CAD build for the part. Positions are in the model's coordinates, mm. Coordinates: 2 decimals unless noted, no trailing zeros. Loops run counter-clockwise (first coordinate to the right, second up) from the corner with the lowest first, then second, coordinate; pieces in that order, holes last. Notation, with made-up numbers: (32, -31.5) -> (79, -31.5) arc R14 ccw to (79, -14.5) -> close; hole circle Ø6 at (54.25, 51). An arc over 180 degrees is marked (long way). Write item = value, one per line. Start each with the question number.
(1) Band-saw the part on A-A (x = 95.45). Write the cut outline in (y, z) (3 decimals).
(2) Drill centre lines: line 1 (X direction, y = -3.75, z = 15); line 2 (Z direction, x = 95.45, y = -2.75); line 3 (Z direction, x = -50, y = -7.5). Where is each one in solid material? Low to high. Write a range as from..to.
(3) Flat gauge pin, fed straight in: P1, Ø6, axis at x = -81, z = -16.5, coming from the +Y side. Where does the tip first touch, or does it go through?
```python
from build123d import *

# Parameters (mm, degrees)
SKETCH1_W             = 240.9
SKETCH1_H             = 50.8
BOSS_EXTRUDE1_DEPTH   = 9.525
M3X0_5_TAPPED_HOLE1_D = 2.5
M5_CLEARANCE_HOLE1_D  = 5.5


with BuildPart() as part:
    # Sketch1 → Boss-Extrude1 (new body)
    with BuildSketch(Plane(origin=(0, 0, 0), x_dir=(1, 0, 0), z_dir=(0, 1, 0))):
        Rectangle(SKETCH1_W, SKETCH1_H)
    extrude(amount=-BOSS_EXTRUDE1_DEPTH)

    # M3x0.5 Tapped Hole1 (through all)
    with Locations(Plane(origin=(0, 0, 0), x_dir=(1, 0, 0), z_dir=(0, 1, 0))):
        with Locations((-50, 15), (-50, -15), (50, -15), (50, 15)):
            Hole(M3X0_5_TAPPED_HOLE1_D / 2)

    # M5 Clearance Hole1 (through all)
    with Locations(Plane(origin=(0, 0, 0), x_dir=(1, 0, 0), z_dir=(0, 1, 0))):
        with Locations((95.45, 15), (-95.45, 15), (-95.45, -15), (95.45, -15)):
            Hole(M5_CLEARANCE_HOLE1_D / 2)


solid = part.part
```
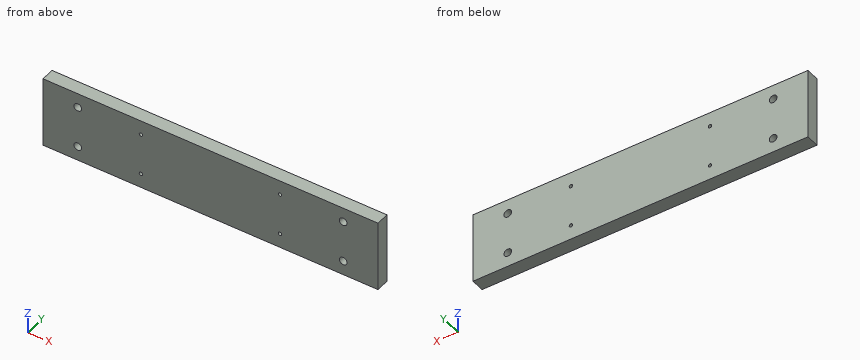
Findings below:
q1.outline = (-9.525, -25.4) -> (0, -25.4) -> (0, -17.75) -> (-9.525, -17.75) -> close; (-9.525, -12.25) -> (0, -12.25) -> (0, 12.25) -> (-9.525, 12.25) -> close; (-9.525, 17.75) -> (0, 17.75) -> (0, 25.4) -> (-9.525, 25.4) -> close
q2.line_1 = -120.45..-98.2, -92.7..-51.25, -48.75..48.75, 51.25..92.7, 98.2..120.45
q2.line_2 = -25.4..-17.75, -12.25..12.25, 17.75..25.4
q2.line_3 = -25.4..-16.25, -13.75..13.75, 16.25..25.4
q3.P1 = 0
